The model under review builds one solid part; all positions refer to its coordinate system, in mm. A direction names the side the tool comes from. Give positions to 0.01 mm unless a question says otherwise; leave off trailing zeros. Order: outer loops, then holes, each group sorted by start corner. A loop starts at its lowest first (then second) coordinate and runs counter-clockwise, first axis right, second up. Notation, with made-up numbers: (27, 60.25) - (49, 60.25) arc R34 ccw to (49, 91.25) - close; hole circle Ø2 at (20, -20). An arc over 180 degrees is marked (long way). Use CSV: the item, a comma, the result in double quotes. Start each with the question number.
```python
from build123d import *

# Parameters (mm, degrees)
F0_W     = 120
F0_H     = 315
F1_DEPTH = 60
F2_W     = 100
F2_H     = 285
F3_DEPTH = 30
F4_T     = -2.5


with BuildPart() as f1:
    # F0 (on Front) → F1 (new body)
    with BuildSketch(Plane.XZ):
        with Locations((60, 157.5)):
            Rectangle(F0_W, F0_H)
    extrude(amount=F1_DEPTH)

    # F2 (on face) → F3 (cut)
    with BuildSketch(Plane.XZ.offset(60)):
        with Locations((120, 157.5)):
            Rectangle(F2_W, F2_H)
    extrude(amount=-F3_DEPTH, mode=Mode.SUBTRACT)

    # F4
    f4_openings = [f1.faces().sort_by_distance(p)[0] for p in [
        (95, -45, 300),
        (70, -45, 157.5),
        (95, -30, 157.5),
        (95, -45, 15),
    ]]
    offset(amount=F4_T, openings=f4_openings)


solid = f1.part
```
1. Clearance check with flat-ended pins moving along their axes: pin 1 (9 mm diameter, centred on x = 89, y = -42.5, fed in from -Z); pin 2 (1.2 mm diameter, centred on y = -58.5, z = 122, fed in from +X); pin 3 (2 mm diameter, centred on x = 118.5, z = 176, fed in from -Y). State where each tip first meets the part, or that it passes through.
2. Consider section C-C (y = -6.5). Give the boundary of the cut face in (x, z).
3. Tool access review of faces 5 (the face through (102, -58, 300)), 6 (the face through (32, -60, 160)), 7 (the face through (2.5, -30, 155)): name each direction out of +Z, -Z, +X, -X, +Y, -Y from which nothing blocks a thin tool from reaching the whole face with its end or side.
4. Consider section A-A (x = 14.5). Give the boundary of the cut face in (y, z).
5. Consider section B-B (z = 250). Give the boundary of the cut face in (x, y).
6. Consider section D-D (y = -41). Give the boundary of the cut face in (x, z).
7. Mouldability with a two-part tool opening along Z and no side actions: class faces 1 (the face through (59, -30, 2.5)), 2 (the face through (0, -30, 155)), 3 (the face through (59, -30, 315)), 4 (the face through (59, -30, 0)) as pulls with the +Z half, pulls with the -Z half, needs draft (parallel to the pull), parting line crosses it, or undercut.
8. To check wall thickness, follow L1, parallel to X at y = -16.5, z = 274; L2, parallel to Z at x = 45.5, y = -55; L3, parallel to Y at x = 49, z = 296. State the ranges of each line that lie inside material, in increasing order. Write a range as [from, to].
Answers follow:
1,pin 1,"stops at z = 0"
1,pin 2,"stops at x = 70"
1,pin 3,"stops at y = -30"
2,outline,"(0, 0) - (120, 0) - (120, 315) - (0, 315) - close; hole (2.5, 2.5) - (117.5, 2.5) - (117.5, 312.5) - (2.5, 312.5) - close"
3,face 5,"+X, -Y"
3,face 6,"+Z, -Z, +X, -X, -Y"
3,face 7,"none"
4,outline,"(-60, 0) - (0, 0) - (0, 315) - (-60, 315) - close; hole (-57.5, 2.5) - (-2.5, 2.5) - (-2.5, 312.5) - (-57.5, 312.5) - close"
5,outline,"(0, -60) - (70, -60) - (70, -57.5) - (2.5, -57.5) - (2.5, -2.5) - (117.5, -2.5) - (117.5, -30) - (120, -30) - (120, 0) - (0, 0) - close"
6,outline,"(0, 0) - (120, 0) - (120, 15) - (117.5, 15) - (117.5, 2.5) - (2.5, 2.5) - (2.5, 312.5) - (117.5, 312.5) - (117.5, 300) - (120, 300) - (120, 315) - (0, 315) - close"
7,face 1,"undercut"
7,face 2,"needs draft"
7,face 3,"pulls with the +Z half"
7,face 4,"pulls with the -Z half"
8,L1,"x = [0, 2.5], [117.5, 120]"
8,L2,"z = [0, 2.5], [312.5, 315]"
8,L3,"y = [-60, -57.5], [-2.5, 0]"
